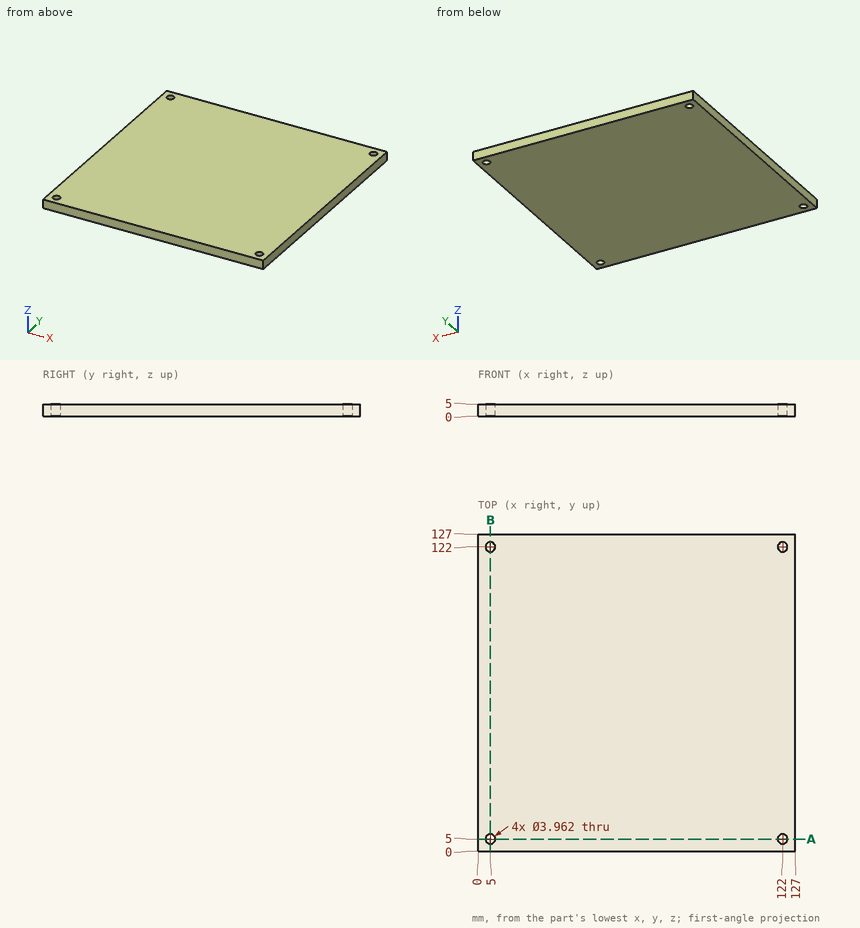
Drawing for the job (mm, zero at the part's lowest x, y, z). Round coordinates to 2 decimals unless told otherwise and drop trailing zeros. Loops run counter-clockwise (first coordinate to the right, second up) from the corner with the lowest first, then second, coordinate; pieces in that order, holes last.
1. Band-saw the part on A-A, the plane y = 5. List the corners of the cut face in (x, z).
Check values:
outline: (0, 0) - (3.02, 0) - (3.02, 5) - (0, 5) - close; (6.98, 0) - (120.02, 0) - (120.02, 5) - (6.98, 5) - close; (123.98, 0) - (127, 0) - (127, 5) - (123.98, 5) - close
2. Drop a flat-ended pin along its axis: P1, Ø2.5, axis at x = 122, y = 122, coming from the -Z side. Give the stop position or say it passes through.
Check values:
P1: passes through
3. Wall check: probe 1 along Y at (x, z) = (5, 1.25). Give the ranges that are in metal, low to high.
Check values:
probe 1: y = 0 to 3.02, 6.98 to 120.02, 123.98 to 127
